Design review of the part built by this model. Coordinates are the model's own, in mm. A direction names the side the tool comes from. Round coordinates to 2 decimals unless told otherwise and drop trailing zeros. Order: outer loops, then holes, each group sorted by start corner. A loop starts at its lowest first (then second) coordinate and runs counter-clockwise, first axis right, second up.
from build123d import *

# Parameters (mm, degrees)
SKETCH_W        = 30
SKETCH_H        = 27
PAD_DEPTH       = 2
SKETCH002_W     = 11
SKETCH002_H     = 27
PAD001_DEPTH    = 28
SKETCH001_R     = 1.5
POCKET001_DEPTH = 2.001
POCKET_DEPTH    = 20.501
POCKET002_DEPTH = 28.001
FILLET_R        = 6
FILLET001_R     = 5
FILLET002_R     = 1
SKETCH005_R     = 1.5
POCKET003_DEPTH = 8
SKETCH006_W     = 7.5
SKETCH006_H     = 4
PAD002_DEPTH    = 15
POCKET004_DEPTH = 4


with BuildPart() as part:
    # Sketch → Pad (new body)
    with BuildSketch(Plane.XY):
        with Locations((15, 13.5)):
            Rectangle(SKETCH_W, SKETCH_H)
    extrude(amount=PAD_DEPTH)

    # Sketch002 (on Face6 of Pad) → Pad001 (join)
    with BuildSketch(Plane.XY.offset(2)):
        with Locations((15, 13.5)):
            Rectangle(SKETCH002_W, SKETCH002_H)
    extrude(amount=PAD001_DEPTH)

    # Sketch001 (on Face6 of Pad) → Pocket001 (cut, through all)
    with BuildSketch(Plane.XY.offset(2)):
        with Locations((3.5, 3.5)):
            Circle(SKETCH001_R)
        with Locations((26.5, 3.5)):
            Circle(SKETCH001_R)
        with Locations((23, 23.5)):
            Circle(SKETCH001_R)
        with Locations((7, 23.5)):
            Circle(SKETCH001_R)
        Polygon((0, 0), (0, 27), (2.5, 27), align=None)
        Polygon((30, 0), (30, 27), (27.5, 27), align=None)
        with BuildLine():
            ThreePointArc((10, 8), (15, 3), (20, 8))
            Line((20, 8), (20, 11))
            ThreePointArc((20, 11), (15, 16), (10, 11))
            Line((10, 8), (10, 11))
        make_face()
    extrude(amount=-POCKET001_DEPTH, mode=Mode.SUBTRACT)

    # Sketch003 (on Face11 of Pad001) → Pocket (cut, through all)
    with BuildSketch(Plane.YZ.offset(20.5)):
        Polygon((0, 30), (18, 30), (0, 2), align=None)
    extrude(amount=-POCKET_DEPTH, mode=Mode.SUBTRACT)

    # Sketch004 (on Face21 of Pocket) → Pocket002 (cut, through all)
    with BuildSketch(Plane(origin=(0, 0, 2), x_dir=(1, 0, 0), z_dir=(0, 0, -1))):
        with BuildLine():
            ThreePointArc((10, -11), (15, -16), (20, -11))
            Line((20, -11), (20, -8))
            ThreePointArc((20, -8), (15, -3), (10, -8))
            Line((10, -11), (10, -8))
        make_face()
    extrude(amount=-POCKET002_DEPTH, mode=Mode.SUBTRACT)

    # Fillet
    fillet_edges = [part.edges().sort_by_distance(p)[0] for p in [
        (27.5, 27, 1),
        (2.5, 27, 1),
    ]]
    fillet(fillet_edges, radius=FILLET_R)

    # Fillet001
    fillet001_edges = [part.edges().sort_by_distance(p)[0] for p in [
        (30, 0, 1),
        (0, 0, 1),
    ]]
    fillet(fillet001_edges, radius=FILLET001_R)

    # Fillet002
    fillet002_edges = [part.edges().sort_by_distance(p)[0] for p in [
        (20.5, 27, 16),
        (9.5, 27, 16),
        (20.5, 9, 16),
        (9.5, 9, 16),
    ]]
    fillet(fillet002_edges, radius=FILLET002_R)

    # Sketch005 (on Face19 of Pocket002) → Pocket003 (cut)
    with BuildSketch(Plane.XY.offset(30)):
        with Locations((15, 22.5)):
            Circle(SKETCH005_R)
    extrude(amount=-POCKET003_DEPTH, mode=Mode.SUBTRACT)

    # Sketch006 (on Face1 of Pocket003) → Pad002 (join)
    with BuildSketch(Plane.XY.offset(2)):
        with Locations((5.75, 13.5)):
            Rectangle(SKETCH006_W, SKETCH006_H)
        with Locations((24.25, 13.5)):
            Rectangle(SKETCH006_W, SKETCH006_H)
    extrude(amount=PAD002_DEPTH)

    # Sketch007 (on Face14 of Pad002) → Pocket004 (cut)
    with BuildSketch(Plane.XZ.offset(-11.5)):
        Polygon((2, 2), (9.5, 17), (2, 17), align=None)
        Polygon((20.5, 17), (28, 2), (28, 17), align=None)
    extrude(amount=-POCKET004_DEPTH, mode=Mode.SUBTRACT)


solid = part.part
1) For faces 1 (the face through (23, 11.5, 8)), 2 (the face through (15, 16, 14)), 3 (the face through (23, 15.5, 8)), 4 (the face through (9.79, 3.2, 6.43)), 5 (the face through (13.89, 23.51, 26.06)), list the 3-axis set-ups (+Z, -Z, +X, -X, +Y, -Y) from which the entire face can be reached by the end or side of a thin tool; tool diameter is ignored.
Results:
face 1: +Z, +X, -Y
face 2: +Z, -Z
face 3: +Z, +X, +Y
face 4: +Z, -X, -Y
face 5: +Z
2) The part is to be moulded in two halves that separate along Y. For faces 6 (the face through (25, 3.57, 1.01)), 7 (the face through (15.063, 16.695, 27.97)), 8 (the face through (15, 27, 15)), say which applies: released by +Y, released by -Y, zero draft, split by the parting line, or undercut.
Results:
face 6: undercut
face 7: released by -Y
face 8: released by +Y
3) Take a section at C-C on x = 23. Give the boundary of the cut face in (y, z), plus the area to 3 significant figures.
Results:
outline: (0, 0) - (22, 0) - (22, 2) - (15.5, 2) - (15.5, 12) - (11.5, 12) - (11.5, 2) - (0, 2) - close; (25, 0) - (26.92, 0) - (26.92, 2) - (25, 2) - close
area: 87.8 mm2
4) Take a section at D-D on x = 15. Give the boundary of the cut face in (y, z).
Results:
outline: (0, 0) - (3, 0) - (3, 6.67) - (0, 2) - close; (16, 0) - (27, 0) - (27, 30) - (24, 30) - (24, 22) - (21, 22) - (21, 30) - (18, 30) - (16, 26.89) - close
5) To check wall thickness, follow line 1 along X through (y, z) = (24.5, 1); line 2 along X through (y, z) = (10, 3); line 3 along X through (y, z) = (22.5, 21). State the ranges of each line that lie inside material, in increasing order.
Results:
line 1: x = 3.1 to 5.88, 8.12 to 21.88, 24.12 to 26.9
line 2: x = 9.5 to 10, 20 to 20.5
line 3: x = 9.5 to 20.5
6) Clearance check with flat-ended pins moving along their axes: P1, Ø8, axis at x = 25.5, y = 11, coming from the +Z side; P2, Ø12, axis at x = 24.5, y = 8.5, coming from the +Z side; P3, Ø12, axis at y = 15.5, z = 9, coming from the +X side. State where each tip first meets the part, or that it passes through.
Results:
P1: stops at z = 14.94
P2: stops at z = 21.28
P3: stops at x = 27.5
7) Take a section at B-B on x = 3.75. Give the boundary of the cut face in (y, z).
Results:
outline: (0.31, 0) - (2.02, 0) - (2.02, 2) - (0.31, 2) - close; (4.98, 0) - (25.27, 0) - (25.27, 2) - (15.5, 2) - (15.5, 5.5) - (11.5, 5.5) - (11.5, 2) - (4.98, 2) - close
8) Take a section at A-A on y = 22.5. Give the boundary of the cut face in (x, z), plus the area to 3 significant figures.
Results:
outline: (2.16, 0) - (5.88, 0) - (5.88, 2) - (2.16, 2) - close; (8.12, 0) - (21.88, 0) - (21.88, 2) - (20.5, 2) - (20.5, 30) - (16.5, 30) - (16.5, 22) - (13.5, 22) - (13.5, 30) - (9.5, 30) - (9.5, 2) - (8.12, 2) - close; (24.12, 0) - (27.84, 0) - (27.84, 2) - (24.12, 2) - close
area: 326 mm2
